from build123d import *

# Parameters (mm, degrees)
F1_DEPTH = 63.5
F2_DEPTH = 25.4
F3_DEPTH = 25.4


# Not quite as in the source:
# - a feature names something its author has since deleted; it is built from what else it names


with BuildPart() as f1:
    # F0 (on Front) → F1 (new body, symmetric)
    with BuildSketch(Plane.XZ):
        Polygon((28.5749990565, 9.525), (-41.275, 9.525), (-41.275, -9.525), (41.275, -9.525), (41.275, 9.525), align=None)
    extrude(amount=F1_DEPTH, both=True)

    # F0 (on Front) → F2 (join, symmetric)
    with BuildSketch(Plane.XZ):
        with BuildLine():
            add(Edge.make_bspline(
                [(-41.275, 9.525), (-23.8584346144, 27.5869780948), (3.0069667421, 45.9865968148), (31.8262, 53.1677247911)],
                knots=[0, 0, 0, 0, 84.5177049164, 84.5177049164, 84.5177049164, 84.5177049164], degree=3))
            Line((-41.275, 9.525), (28.5749990565, 9.525))
            Line((28.5749990565, 9.525), (28.5749990565, 25.7647229111))
            ThreePointArc((28.5749990565, 25.7647229111), (29.8677699589, 34.2739896946), (33.6294204286, 42.0153631867))
            Line((33.6294204286, 42.0153631867), (31.8262, 42.0153631867))
            Line((31.8262, 42.0153631867), (31.8262, 53.1677247911))
        make_face()
    extrude(amount=F2_DEPTH, both=True)

    # F0 (on Front) → F3 (join, symmetric)
    with BuildSketch(Plane.XZ):
        Polygon((31.8262, 70.5903631867), (31.8262, 53.1677247911), (31.8262, 42.0153631867), (33.6294204286, 42.0153631867), (82.6262, 42.0153631867), (82.6262, 70.5903631867), align=None)
    extrude(amount=F3_DEPTH, both=True)

    # F0 (on Front) → F6 (revolve)
    with BuildSketch(Plane.XZ):
        Polygon((31.8262, 70.5903631867), (31.8262, 53.1677247911), (31.8262, 42.0153631867), (33.6294204286, 42.0153631867), (82.6262, 42.0153631867), (82.6262, 70.5903631867), align=None)
    revolve(axis=Axis((82.6262, 0, 56.3028631867), (0, 0, 1)))


solid = f1.part
Can you work these out from the model? Positions are in its coordinate system, mm. A direction names the side the tool comes from. Coordinates: 2 decimals unless noted, no trailing zeros. Loops run counter-clockwise (first coordinate to the right, second up) from the corner with the lowest first, then second, coordinate; pieces in that order, holes last. Notation, with made-up numbers: M 77,63 L 127,63 A28 cw 127,85 Z; hole C 79,4 d3. An arc over 180 degrees is marked long. Answer as CSV lines item,"result". Start each with the question number.
1. For faces 1 (the face through (7, -25.4, 27)), 2 (the face through (7, 25.4, 27)), 3 (the face through (28.575, 0, 18)), 4 (the face through (31.826, 0, 62)), which set-ups out of +Z, -Z, +X, -X, +Y, -Y let a thin tool reach every point of the face, with its end or its side?
2. Suppose I cut it at A-A, the plane y = 29.5. List the corners of the cut face in (x, z) for me (3 decimals).
3. Suppose I cut it at D-D, the plane x = 89.5. List the corners of the cut face in (y, z) for me, plus the area to 3 significant figures.
4. For pin 1 Ø5.5 at (y, z) = (-5.5, 1.5) entering from +X (3 decimals); pin 2 Ø8 at (x, y) = (6, -48) entering from +Z (3 decimals); pin 3 Ø14 at (y, z) = (-9, 65) entering from -X, each with a flat end and sliding along its axis, tell me the tip position at first contact or that it passes through.
5. Suppose I cut it at B-B, the plane y = -33.5. List the corners of the cut face in (x, z) for me (3 decimals).
6. Suppose I cut it at C-C, the plane z = -1. List the corners of the cut face in (x, y) for me (3 decimals).
7. If I drill on probe 1 along Z at (x, y) = (34, 3) (3 decimals); probe 2 along Z at (x, y) = (55.5, 23); probe 3 along X at (y, z) = (46.5, -5.5) (3 decimals), over which ranges is the centre line in solid material (lowest first)? Write a range as [from, to].
8. Thinking about a two-plate mould opening in Z: for faces 5 (the face through (41.275, -1, 0)), 6 (the face through (82, -1, 70.59)), 7 (the face through (29.832, -0.356, 34.158)), which applies, +Z half, -Z half, draft (parallel to the pull), parting line (faces both ways), or undercut?
Output:
1,face 1,"+Z, -X, -Y"
1,face 2,"+Z, -X, +Y"
1,face 3,"+X, +Y, -Y"
1,face 4,"+Z, -X, +Y, -Y"
2,outline,"M -41.275,-9.525 L 41.275,-9.525 L 41.275,9.525 L -41.275,9.525 Z; M 41.269,42.015 L 123.983,42.015 L 123.983,70.59 L 41.269,70.59 Z"
3,outline,"M -50.33,42.02 L 50.33,42.02 L 50.33,70.59 L -50.33,70.59 Z"
3,area,"2,880 mm^2"
4,pin 1,"stops at x = 41.275"
4,pin 2,"stops at z = 9.525"
4,pin 3,"stops at x = 31.83"
5,outline,"M -41.275,-9.525 L 41.275,-9.525 L 41.275,9.525 L -41.275,9.525 Z; M 44.437,42.015 L 120.815,42.015 L 120.815,70.59 L 44.437,70.59 Z"
6,outline,"M -41.275,-63.5 L 41.275,-63.5 L 41.275,63.5 L -41.275,63.5 Z"
7,probe 1,"z = [-9.525, 9.525], [42.015, 70.59]"
7,probe 2,"z = [42.02, 70.59]"
7,probe 3,"x = [-41.275, 41.275]"
8,face 5,"draft"
8,face 6,"+Z half"
8,face 7,"undercut"
